```python
from build123d import *

# Parameters (mm, degrees)
BOSS_EXTRUDE1_DEPTH = 63.246
SKETCH2_R           = 11.953875
BOSS_EXTRUDE2_DEPTH = 5.08


with BuildPart() as part:
    # Sketch1 → Boss-Extrude1 (new body)
    with BuildSketch(Plane.XY):
        with BuildLine():
            Line((-7.874, -23.606125), (7.874, -23.606125))
            ThreePointArc((7.874, -23.606125), (10.886228439, -19.550079279), (11.953875, -14.611946243))
            Line((11.953875, -14.611946243), (11.953875, 0))
            ThreePointArc((11.953875, 0), (0, 11.953875), (-11.953875, 0))
            Line((-11.953875, 0), (-11.953875, -14.611946243))
            ThreePointArc((-11.953875, -14.611946243), (-10.886228439, -19.550079279), (-7.874, -23.606125))
        make_face()
    extrude(amount=BOSS_EXTRUDE1_DEPTH)

    # Sketch2 → Boss-Extrude2 (add)
    with BuildSketch(Plane.XY.offset(63.246)):
        Circle(SKETCH2_R)
    extrude(amount=BOSS_EXTRUDE2_DEPTH)

    # Sketch3 → Revolve1 (revolve)
    with BuildSketch(Plane(origin=(0, 0, 0), x_dir=(0, 0, -1), z_dir=(1, 0, 0)), mode=Mode.PRIVATE) as revolve1_sk:
        with BuildLine():
            Line((-74.2696, 0), (-68.326, 0))
            Line((-68.326, 0), (-68.326, 11.953875))
            ThreePointArc((-68.326, 11.953875), (-70.242328664, 11.415006517), (-72.009, 10.49763681))
            Line((-72.009, 10.49763681), (-71.2978, 8.921350892))
            ThreePointArc((-71.2978, 8.921350892), (-73.507109881, 4.701651225), (-74.2696, 0))
        make_face()
    revolve(revolve1_sk.sketch.rotate(Axis((0, 0, 74.2696), (0, 0, -1)), 180), axis=Axis((0, 0, 74.2696), (0, 0, -1)))


solid = part.part
```
The listing builds one solid part. Answer for the finished solid, in the listing's coordinates (mm). Give positions to 0.01 mm unless a question says otherwise; leave off trailing zeros. Order: outer loops, then holes, each group sorted by start corner. A loop starts at its lowest first (then second) coordinate and runs counter-clockwise, first axis right, second up. Notation, with made-up numbers: (74.25, 29.5) - (95.25, 29.5) arc R32 ccw to (95.25, 55.5) - close; hole circle Ø9 at (17.25, 31.25). An arc over 180 degrees is marked (long way). Use one line per item in the form item = value. Start each with the question number.
(1) A cutting plane is placed at A-A, the plane z = 20.5. Write down the section's boundary in (x, y), then the cut area to 3 significant figures.
(2) A cutting plane is placed at B-B, the plane y = -16.5. Write down the section's boundary in (x, z), then the cut area to 3 significant figures.
(3) Consider line 1 (Z direction, x = -1.5, y = -15.5); line 2 (Y direction, x = 0.5, z = 4); line 3 (Y direction, x = -6.5, z = 40.5). Determine where each line is inside the solid, lowest interval first. Write a range as from..to.
(4) Flat-ended cylindrical pins translate along their axes: pin 1 Ø1 at (x, y) = (-4, 0.5) entering from +Z; pin 2 Ø12 at (x, z) = (7.5, 28) entering from +Y; pin 3 Ø2 at (x, y) = (-9, 6.5) entering from +Z. Find the tip coordinate at first contact, or state that the pin passes through.
Ans:
q1.outline = (-11.95, -14.61) arc R11.95 ccw to (-7.87, -23.61) - (7.87, -23.61) arc R11.95 ccw to (11.95, -14.61) - (11.95, 0) arc R11.95 ccw to (-11.95, 0) - close
q1.area = 766 mm^2
q2.outline = (-11.8, 0) - (11.8, 0) - (11.8, 63.25) - (-11.8, 63.25) - close
q2.area = 1,490 mm^2
q3.line_1 = 0..63.25
q3.line_2 = -23.61..11.94
q3.line_3 = -23.61..10.03
q4.pin_1 = 73.84
q4.pin_2 = 11.86
q4.pin_3 = 72.01
